Check sheet for the modelled part. Datum: model origin and axes. Units: mm. Round coordinates to 2 decimals unless told otherwise and drop trailing zeros. Write each loop counter-clockwise with the first axis right and the second up, starting at its lowest first coordinate (ties: lowest second). Pieces come first, ordered by that corner, then holes. Notation, with made-up numbers: M 76,-23 L 108,-23 A11 cw 108,-18 Z; hole C 19,-38.75 d7. An arc over 180 degrees is marked long. Answer in a Markdown table with one row per item.
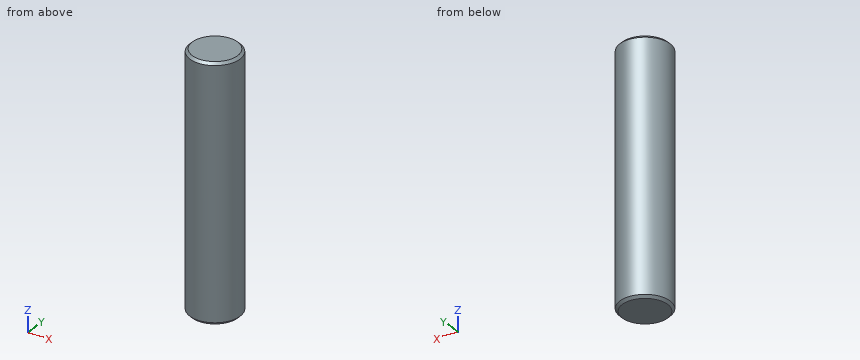
```python
from build123d import *

# Parameters (mm, degrees)
F0_R     = 10
F1_DEPTH = 100
F2_SIZE  = 1
F3_SIZE  = 1


with BuildPart() as f1:
    # F0 (on Top) → F1 (new body)
    with BuildSketch(Plane.XY):
        with Locations((-11.811228, 7.31832)):
            Circle(F0_R)
    extrude(amount=F1_DEPTH)

    # F2
    f2_edges = [f1.edges().sort_by_distance(p)[0] for p in [
        (-21.811228, 7.31832, 100),
    ]]
    chamfer(f2_edges, length=F2_SIZE)

    # F3
    f3_edges = [f1.edges().sort_by_distance(p)[0] for p in [
        (-21.811228, 7.31832, 0),
    ]]
    chamfer(f3_edges, length=F3_SIZE)


solid = f1.part
```
1. Section check A-A, the plane z = 12. Record the cut outline in (x, y), and give its area (3 significant figures).
Found:
| item | result |
|---|---|
| outline | C -11.81,7.32 d20 |
| area | 314 mm2 |
2. Scan lines: L1, parallel to Y at x = -11.25, z = 24; L2, parallel to Y at x = -20.5, z = 10.5; L3, parallel to X at y = 4, z = 20.5. Record each from-to range of solid material in increasing order.
Found:
| item | result |
|---|---|
| L1 | y = -2.67 to 17.3 |
| L2 | y = 2.37 to 12.27 |
| L3 | x = -21.24 to -2.38 |
3. Go/stop test with flat-tipped pins: pin 1 (1.5 mm diameter, centred on x = -14.5, z = 12.5, fed in from +Y); pin 2 (2 mm diameter, centred on y = 1.5, z = 78, fed in from +X); pin 3 (1 mm diameter, centred on x = -4, z = 16, fed in from +Y). Record where each tip stops, or that it passes through.
Found:
| item | result |
|---|---|
| pin 1 | stops at y = 17.13 |
| pin 2 | stops at x = -3.05 |
| pin 3 | stops at y = 14.14 |
